CAD build for the part. Positions are in the model's coordinates, mm. Give positions to 0.01 mm unless a question says otherwise; leave off trailing zeros. Loops run counter-clockwise (first coordinate to the right, second up) from the corner with the lowest first, then second, coordinate; pieces in that order, holes last. Notation, with made-up numbers: M 44,-32.5 L 72,-32.5 A28 ccw 72,-14.5 Z; hole C 15.25,39 d5. An arc over 180 degrees is marked long. One line per question, with ' | ' between items.
```python
from build123d import *

# Parameters (mm, degrees)
BOSS_EXTRUDE1_DEPTH = 1
SKETCH3_R           = 1.755
CUT_EXTRUDE2_DEPTH  = 171.729965471


with BuildPart() as part:
    # Sketch1 → Boss-Extrude1 (new body)
    with BuildSketch(Plane(origin=(0, 0, 0), x_dir=(1, 0, 0), z_dir=(0, 1, 0))):
        with BuildLine():
            Line((-24.22232668, 167.255131133), (-7.949423814, 64.512066011))
            ThreePointArc((-7.949423814, 64.512066011), (0, 65), (7.949423814, 64.512066011))
            Line((7.949423814, 64.512066011), (24.22232668, 167.255131133))
            ThreePointArc((24.22232668, 167.255131133), (0, 169), (-24.22232668, 167.255131133))
        make_face()
    extrude(amount=BOSS_EXTRUDE1_DEPTH)

    # Sketch3 → Cut-Extrude2 (cut, through all)
    with BuildSketch(Plane.XZ):
        with Locations(Location((0.196844211, -82.845225749, 0), (0, 0, 270))):
            Circle(SKETCH3_R)
        with Locations(Location((0.315646263, -132.845084609, 0), (0, 0, 270))):
            Circle(SKETCH3_R)
    extrude(amount=-CUT_EXTRUDE2_DEPTH, mode=Mode.SUBTRACT)


solid = part.part
```
Item 1: Mould opens along X. For faces 1 (the flat face through (-16.2, 0.5, -116.6)), 2 (the flat face through (0, 0, -129)), 3 (the cylindrical face through (0.72, 0.49, -84.52)) say: pulls with the +X half, pulls with the -X half, needs draft (parallel to the pull), parting line crosses it, or undercut.
Conclusion:
face 1: pulls with the -X half | face 2: needs draft | face 3: undercut
Item 2: Saw through at A-A on y = 0.15. Give the cut face in (x, z) (3 decimals).
Conclusion:
outline: M -24.222,-167.255 A169 ccw 24.222,-167.255 L 7.949,-64.512 A65 cw -7.949,-64.512 Z; hole C 0.197,-82.845 d3.51; hole C 0.316,-132.845 d3.51
Item 3: Drop a flat-ended pin along its axis: P1, Ø12, axis at x = 14.5, z = -83.5, coming from the +Y side. Give the stop position or say it passes through.
Conclusion:
P1: y = 1
Item 4: Saw through at C-C on x = 20. Give the cut face in (y, z).
Conclusion:
outline: M 0,-167.81 L 1,-167.81 L 1,-140.6 L 0,-140.6 Z
Item 5: Drill centre lines: line 1 along Z through (x, y) = (-1, 0.1); line 2 along X through (y, z) = (0.4, -77); line 3 along X through (y, z) = (0.2, -89.5). Where is each one in solid material? Low to high. Write a range as [from, to].
Conclusion:
line 1: [-169, -134.01], [-131.68, -84.13], [-81.56, -64.99] | line 2: [-9.93, 9.93] | line 3: [-11.91, 11.91]
Item 6: Saw through at B-B on z = -158. Give the cut face in (x, y), and give its area (3 significant figures).
Conclusion:
outline: M -22.76,0 L 22.76,0 L 22.76,1 L -22.76,1 Z | area: 45.5 mm²
